```python
from build123d import *

# Parameters (mm, degrees)
PAD_DEPTH = 10


with BuildPart() as part:
    # Sketch001 → Pad (new body)
    with BuildSketch(Plane.XY):
        with BuildLine():
            ThreePointArc((24, -6), (32.130235, -2.582329), (38, 4))
            ThreePointArc((38, 4), (41.881212, 13.836388), (44.8, 24))
            Line((-36, 24), (44.8, 24))
            ThreePointArc((-36, 24), (-27.362437, 6.310051), (-12, -6))
            Line((-12, -6), (24, -6))
        make_face()
    extrude(amount=PAD_DEPTH)


solid = part.part
```
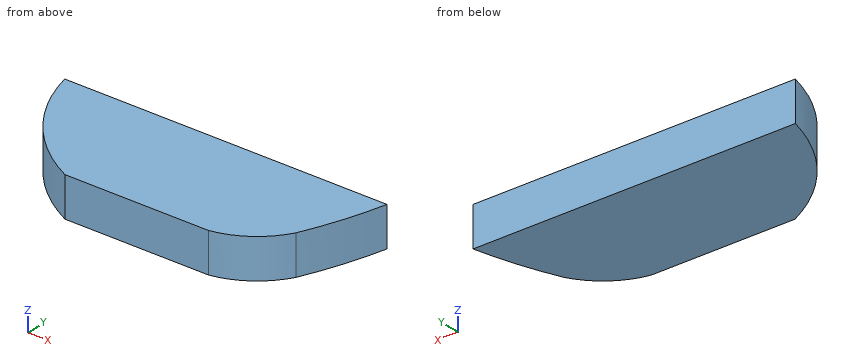
Check sheet for the modelled part. Datum: model origin and axes. Units: mm. Round coordinates to 2 decimals unless told otherwise and drop trailing zeros. Order: outer loops, then holes, each group sorted by start corner. A loop starts at its lowest first (then second) coordinate and runs counter-clockwise, first axis right, second up. Notation, with made-up numbers: (-29.75, 27) -> (-16.75, 27) arc R27 ccw to (-16.75, 62) -> close; hole circle Ø2 at (-30, 88). An arc over 180 degrees is marked (long way). One line per item, written item: value. Start each with the question number.
Q1. Cross-section at B-B (y = 13). Record the boundary of the cut face in (x, z), and give its area (3 significant figures).
Q2. Gauge pin test, flat ends, axial feed: pin 1 Ø3 at (y, z) = (18.5, 7.5) entering from -X; pin 2 Ø2 at (x, z) = (-27, 8.5) entering from -Y; pin 3 Ø2 at (y, z) = (16.5, 4.5) entering from -X. Record the tip position at first contact, or that the pin passes through.
Q3. Cross-section at A-A (z = 9). Record the boundary of the cut face in (x, y), and give its area (3 significant figures).
Q4. Thickness scan on line 1 (Y direction, x = 38, z = 8.25); line 2 (X direction, y = 12.5, z = 4.5); line 3 (X direction, y = 7, z = 2.5). Record the ranges inside material, lowest first.
Q5. Cross-section at C-C (x = -26). Record the boundary of the cut face in (y, z).
Completed:
1. outline: (-31.8, 0) -> (41.59, 0) -> (41.59, 10) -> (-31.8, 10) -> close
1. area: 734 mm²
2. pin 1: stops at x = -34.85
2. pin 2: stops at y = 4.69
2. pin 3: stops at x = -33.92
3. outline: (-36, 24) arc R45 ccw to (-12, -6) -> (24, -6) arc R20 ccw to (38, 4) arc R110 ccw to (44.8, 24) -> close
3. area: 2,000 mm²
4. line 1: y = 4 to 24
4. line 2: x = -31.52 to 41.42
4. line 3: x = -27.9 to 39.3
5. outline: (4.69, 0) -> (24, 0) -> (24, 10) -> (4.69, 10) -> close
